Geometry: final body of the model. Coordinates: model frame, mm. A direction names the side the tool comes from. Give positions to 0.01 mm unless a question says otherwise; leave off trailing zeros. Write each loop counter-clockwise with the first axis right and the second up, starting at its lowest first coordinate (ties: lowest second). Pieces come first, ordered by that corner, then holes. Notation, with made-up numbers: (11.25, 45.5) -> (56.25, 45.5) arc R38 cw to (56.25, 84.5) -> close; hole circle Ø2 at (-22.75, -37.5). An arc over 180 degrees is marked (long way). Answer in a Markdown table with one row per item. Add a question column.
from build123d import *

# Parameters (mm, degrees)
SKETCH2_W           = 15.88
SKETCH2_H           = 12.7
SKETCH2_R           = 3.25
BOSS_EXTRUDE1_DEPTH = 8.255
SKETCH3_R           = 2.97
CUT_EXTRUDE1_DEPTH  = 44.847035248


with BuildPart() as part:
    # Sketch1 → Revolve1 (revolve)
    with BuildSketch(Plane(origin=(0, 0, 0), x_dir=(1, 0, 0), z_dir=(0, 1, 0))):
        Polygon((-40, 8), (-35.2, 8), (-35.2, 6), (-30.6, 6), (-30.6, 8), (-1.732050808, 8), (0, 5), (8.255, 5), (10.655438173, 1.005), (11.122943817, 1.005), (11.122943817, 0.175), (9.112544042, 0.175), (7.264897638, 3.25), (0, 3.25), (-40, 3.25), align=None)
    revolve(axis=Axis((0, 0, 0), (-1, 0, 0)))

    # Sketch2 → Boss-Extrude1 (add)
    with BuildSketch(Plane(origin=(0, 0, 0), x_dir=(0, 0, -1), z_dir=(1, 0, 0))):
        with Locations((-2.86, 0)):
            Rectangle(SKETCH2_W, SKETCH2_H)
        Circle(SKETCH2_R, mode=Mode.SUBTRACT)
    extrude(amount=BOSS_EXTRUDE1_DEPTH)

    # Sketch3 → Cut-Extrude1 (cut, through all)
    with BuildSketch(Plane(origin=(0, 6.35, 0), x_dir=(1, 0, 0), z_dir=(0, 1, 0))):
        with Locations(Location((4.115, -6.99, 0), (0, 0, 270))):
            Circle(SKETCH3_R)
    extrude(amount=-CUT_EXTRUDE1_DEPTH, mode=Mode.SUBTRACT)


solid = part.part
Q1. Contact query for flat-ended pins moving along their axis: pin 1 Ø5 at (x, z) = (-18.5, -5) entering from -Y; pin 2 Ø10 at (x, z) = (-17.5, 7.5) entering from +Y; pin 3 Ø9.5 at (x, z) = (4.115, 6.99) entering from +Y. Output: stop coordinate, or through.
Q2. Pull-direction query (Y, two-part tool) for faces 1 (the conical face through (8.997, -0.11, -0.35)), 2 (the cylindrical face through (-33, 0, 6)), 3 (the flat face through (4, -6.35, 1)), 4 (the flat face through (8.255, 0, 7)); classes: +Y half, -Y half, draft (parallel to the pull), parting line (faces both ways), or undercut.
Q3. Access query for faces 5 (the flat face through (4, 6.35, 1)), 6 (the cylindrical face through (10.89, -0.3, -0.96)), 7 (the cylindrical face through (-16.037, 1.978, 2.579)). Directions: +Z, -Z, +X, -X, +Y, -Y. A direction counts if a zero-diameter tool reaches every point of the face in a straight line with its end or side. Return the directions, or none.
Q4. Line query: probe 1 along X at (y, z) = (0, 6.99) (3 decimals); probe 2 along Z at (x, y) = (-8, 0); probe 3 along X at (y, z) = (-0.75, 7.5) (3 decimals). Output: solid intervals per line, ascending. Write a range as from..to.
Q5. Section B-B on y = -5.5. Count the separate pieces of the cut face and the enclosed holes in it, and give its area (3 significant figures).
Q6. Section A-A on x = -30. Return loops of the section in (y, z).
Checks:
| question | item | result |
|---|---|---|
| 1 | pin 1 | y = -7.6 |
| 1 | pin 2 | y = 7.6 |
| 1 | pin 3 | y = 6.35 |
| 2 | face 1 | undercut |
| 2 | face 2 | parting line |
| 2 | face 3 | -Y half |
| 2 | face 4 | draft |
| 3 | face 5 | +Z, -Z, +X, +Y |
| 3 | face 6 | +X |
| 3 | face 7 | -X |
| 4 | probe 1 | -40..-35.2, -30.6..-1.149, 0..1.145, 7.085..8.255 |
| 4 | probe 2 | -8..-3.25, 3.25..8 |
| 4 | probe 3 | -40..-35.2, -30.6..-1.465, 0..1.189, 7.041..8.255 |
| 5 | separate pieces | 2 |
| 5 | enclosed holes | 1 |
| 5 | area | 527 mm^2 |
| 6 | outline | circle Ø16 at (0, 0); hole circle Ø6.5 at (0, 0) |
